Part model, mm, in its own coordinate system. Give positions to 0.01 mm unless a question says otherwise; leave off trailing zeros. Write each loop counter-clockwise with the first axis right and the second up, starting at its lowest first coordinate (ties: lowest second). Pieces come first, ordered by that corner, then holes.
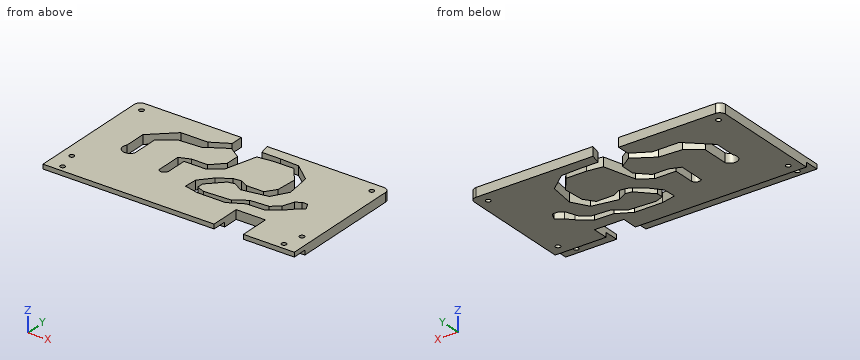
from build123d import *

# Parameters (mm, degrees)
PAD_DEPTH            = 83.675
SKETCH001_R          = 1.58
POCKET_DEPTH         = 377.510907
POCKET_DEPTH_BACK    = 383.510907
SKETCH002_R          = 1.58
POCKET001_DEPTH      = 377.510907
POCKET001_DEPTH_BACK = 383.510907
FILLET_R             = 4
POCKET002_DEPTH      = 0.001
POCKET002_DEPTH_BACK = 6.001
POCKET003_DEPTH      = 10.5


with BuildPart() as part:
    # Sketch → Pad (new body, symmetric)
    with BuildSketch(Plane.YZ):
        Polygon((0, 6), (77.5, 6), (77.5, 0), (0, 0), (0, 3), (-9.6, 3), (-9.6, 6), align=None)
    extrude(amount=PAD_DEPTH, both=True)

    # Sketch001 → Pocket (cut, two sides)
    with BuildSketch(Plane.XY) as pocket_sk:
        with Locations((-73.675, -5.4)):
            Circle(SKETCH001_R)
    pocket = extrude(amount=-POCKET_DEPTH, mode=Mode.SUBTRACT) + extrude(pocket_sk.sketch, amount=POCKET_DEPTH_BACK, mode=Mode.SUBTRACT)

    # Mirrored: Pocket across Sketch001 V_Axis
    add(pocket.mirror(Plane(origin=(0, 0, 0), x_dir=(0, 0, 1), z_dir=(1, 0, 0))), mode=Mode.SUBTRACT)

    # Sketch002 → Pocket001 (cut, two sides)
    with BuildSketch(Plane.XY) as pocket001_sk:
        with Locations((-76.675, 7)):
            Circle(SKETCH002_R)
        with Locations((-76.675, 70.5)):
            Circle(SKETCH002_R)
    pocket001 = extrude(amount=-POCKET001_DEPTH, mode=Mode.SUBTRACT) + extrude(pocket001_sk.sketch, amount=POCKET001_DEPTH_BACK, mode=Mode.SUBTRACT)

    # Mirrored001: Pocket001 across Sketch002 V_Axis
    add(pocket001.mirror(Plane(origin=(0, 0, 0), x_dir=(0, 0, 1), z_dir=(1, 0, 0))), mode=Mode.SUBTRACT)

    # Fillet
    fillet_edges = [part.edges().sort_by_distance(p)[0] for p in [
        (-83.675, 77.5, 3),
        (83.675, 77.5, 3),
    ]]
    fillet(fillet_edges, radius=FILLET_R)

    # Sketch003 → Pocket002 (cut, two sides)
    with BuildSketch(Plane.XY) as pocket002_sk:
        with BuildLine():
            Line((0, 85.498085), (-15.298519, 85.498085))
            Line((-15.298519, 85.498085), (-15.298519, 69.177368))
            Line((-15.298519, 69.177368), (-26.769978, 62.684086))
            Line((-26.769978, 62.684086), (-44.734715, 62.684086))
            Line((-44.734715, 62.684086), (-59.872273, 48.831764))
            Line((-59.872273, 48.831764), (-59.872273, 34.509105))
            ThreePointArc((-59.872273, 34.509105), (-58.127246, 27.428906), (-51.248122, 29.847994))
            Line((-51.248122, 29.847994), (-51.248122, 47.74955))
            Line((-51.248122, 47.74955), (-41.271629, 55.108601))
            Line((-41.271629, 55.108601), (-26.120649, 55.974365))
            Line((-26.120649, 55.974365), (-12.268326, 64.415634))
            Line((-12.268326, 64.415634), (-4.273829, 59.00457))
            Line((-4.273829, 59.00457), (-4.273829, 49.746376))
            Line((-4.273829, 49.746376), (-11.849321, 42.138565))
            Line((-11.849321, 42.138565), (-22.578484, 42.138565))
            Line((-22.578484, 42.138565), (-29.684225, 39.336304))
            Line((-29.684225, 39.336304), (-29.684225, 21.921904))
            ThreePointArc((-29.684225, 21.921904), (-26.450024, 21.191665), (-24.355623, 23.762032))
            Line((-24.355623, 23.762032), (-24.355623, 37.648584))
            Line((-24.355623, 37.648584), (-10.103902, 37.648584))
            Line((-10.103902, 37.648584), (-1.662641, 43.420704))
            Line((-1.662641, 43.420704), (4.266177, 64.735275))
            Line((4.266177, 64.735275), (14.620769, 66.093262))
            Line((14.620769, 66.093262), (27.998238, 66.093262))
            Line((27.998238, 66.093262), (36.006613, 55.757923))
            Line((36.006613, 55.757923), (35.051826, 42.016021))
            Line((35.051826, 42.016021), (30.290104, 35.52275))
            Line((30.290104, 35.52275), (18.682957, 35.52275))
            Line((18.682957, 35.52275), (13.581733, 38.294209))
            Line((13.581733, 38.294209), (8.170669, 37.644886))
            Line((8.170669, 37.644886), (0, 32.382126))
            Line((0, 32.382126), (-6.857254, 24.373747))
            Line((-6.857254, 24.373747), (-7.290145, 15.716045))
            Line((-7.290145, 15.716045), (2.203666, 13.517555))
            Line((2.203666, 13.517555), (20.817725, 13.517555))
            Line((20.817725, 13.517555), (30.746775, 18.903475))
            Line((30.746775, 18.903475), (43.285458, 19.26811))
            Line((43.285458, 19.26811), (51.726704, 25.761387))
            Line((51.726704, 25.761387), (55.560936, 29.718502))
            Line((60.111149, 33.261222), (55.560936, 29.718502))
            Line((57.811371, 38.052417), (60.111149, 33.261222))
            Line((54.002171, 38.084934), (57.811371, 38.052417))
            Line((50.578094, 35.659588), (54.002171, 38.084934))
            Line((47.703377, 28.185322), (50.578094, 35.659588))
            Line((42.337234, 23.969067), (47.703377, 28.185322))
            Line((29.880125, 23.202477), (42.337234, 23.969067))
            Line((21.830915, 17.64469), (29.880125, 23.202477))
            Line((4.007673, 16.686453), (21.830915, 17.64469))
            Line((-1.358464, 18.794577), (4.007673, 16.686453))
            Line((-1.358464, 23.01083), (-1.358464, 18.794577))
            Line((8.223927, 32.78487), (-1.358464, 23.01083))
            Line((12.631821, 33.55146), (8.223927, 32.78487))
            Line((18.9562, 29.910152), (12.631821, 33.55146))
            Line((36.012859, 32.976517), (18.9562, 29.910152))
            Line((42.337234, 43.517147), (36.012859, 32.976517))
            Line((40.037453, 60.382156), (42.337234, 43.517147))
            Line((28.346945, 69.964546), (40.037453, 60.382156))
            Line((15.889835, 70.53949), (28.346945, 69.964546))
            Line((3.432726, 70.53949), (15.889835, 70.53949))
            Line((0, 85.498085), (3.432726, 70.53949))
        make_face()
    extrude(amount=-POCKET002_DEPTH, mode=Mode.SUBTRACT)
    extrude(pocket002_sk.sketch, amount=POCKET002_DEPTH_BACK, mode=Mode.SUBTRACT)

    # Sketch004 → Pocket003 (cut, symmetric)
    with BuildSketch(Plane.XZ):
        Polygon((40.015, 0), (30.265, 0), (30.265, 8), (40.015, 8), (49.765, 8), (49.765, 0), align=None)
    extrude(amount=POCKET003_DEPTH, both=True, mode=Mode.SUBTRACT)


solid = part.part
1) Saw through at B-B (x = 46). Write the cut outline in (y, z).
Check result:
outline: (10.5, 0) - (21.36, 0) - (21.36, 6) - (10.5, 6) - close; (26.85, 0) - (77.5, 0) - (77.5, 6) - (26.85, 6) - close
2) Saw through at D-D (z = 5). State how many separate pieces and enclosed holes the cut face has, and give its area (3 significant figures).
Check result:
separate pieces: 1
enclosed holes: 6
area: 12,200 mm2
3) Saw through at A-A (y = 7). Write the cut outline in (x, z) (3 decimals), and give its area (3 significant figures).
Check result:
outline: (-83.675, 0) - (-78.255, 0) - (-78.255, 6) - (-83.675, 6) - close; (-75.095, 0) - (30.265, 0) - (30.265, 6) - (-75.095, 6) - close; (49.765, 0) - (75.095, 0) - (75.095, 6) - (49.765, 6) - close; (78.255, 0) - (83.675, 0) - (83.675, 6) - (78.255, 6) - close
area: 849 mm2
4) Saw through at C-C (y = -5.4). Write the cut outline in (x, z) (3 decimals).
Check result:
outline: (-83.675, 3) - (-75.255, 3) - (-75.255, 6) - (-83.675, 6) - close; (-72.095, 3) - (30.265, 3) - (30.265, 6) - (-72.095, 6) - close; (49.765, 3) - (72.095, 3) - (72.095, 6) - (49.765, 6) - close; (75.255, 3) - (83.675, 3) - (83.675, 6) - (75.255, 6) - close
5) Drill centre lines: L1, parallel to X at y = 7, z = 2.7 (3 decimals); L2, parallel to X at y = 23, z = 5 (3 decimals); L3, parallel to Y at x = 77, z = 1.75. Where is each one in solid material? Low to high.
Check result:
L1: x = -83.675 to -78.255, -75.095 to 30.265, 49.765 to 75.095, 78.255 to 83.675
L2: x = -83.675 to -29.684, -24.554 to -6.926, -1.358 to 29.587, 48.137 to 83.675
L3: y = 0 to 5.45, 8.55 to 68.95, 72.05 to 77.5
6) Flat gauge pins, fed straight in: P1, Ø0.9, axis at x = -43.5, z = 2, coming from the -Y side; P2, Ø3, axis at x = 62, y = -6.5, coming from the -Z side; P3, Ø16, axis at x = -55.79, y = 31.76, coming from the +Z side. Where does each tip first touch, or does it go through?
Check result:
P1: stops at y = 0
P2: stops at z = 3
P3: stops at z = 6
